Geometry: final body of the model. Coordinates: model frame, mm. A direction names the side the tool comes from. Give positions to 0.01 mm unless a question says otherwise; leave off trailing zeros. Order: outer loops, then holes, each group sorted by start corner. A loop starts at its lowest first (then second) coordinate and runs counter-clockwise, first axis right, second up. Notation, with made-up numbers: (43.25, 72.25) - (72.25, 72.25) arc R28 ccw to (72.25, 90.25) - close; hole circle Ø9 at (-23.75, 35). An arc over 180 degrees is marked (long way). One line per question, with ' | ' between items. Start each with the question number.
from build123d import *

# Parameters (mm, degrees)
SKETCH7_W           = 100
SKETCH7_H           = 14.5
BOSS_EXTRUDE1_DEPTH = 16.5
SKETCH8_R           = 4.75
CUT_EXTRUDE2_DEPTH  = 16
CUT_EXTRUDE3_START  = -2
SKETCH9_W           = 27
SKETCH9_H           = 27
CUT_EXTRUDE3_DEPTH  = 2
CUT_EXTRUDE4_DEPTH  = 2
FILLET1_R           = 3
FILLET2_R           = 3
FILLET3_R           = 0.3


with BuildPart() as part:
    # Sketch7 → Boss-Extrude1 (new body)
    with BuildSketch(Plane(origin=(0, 0, 0), x_dir=(0, 1, 0), z_dir=(0, 0, 1))):
        Rectangle(SKETCH7_W, SKETCH7_H)
    extrude(amount=BOSS_EXTRUDE1_DEPTH)

    # Sketch8 → Cut-Extrude2 (cut)
    with BuildSketch(Plane(origin=(0, 0, 16.5), x_dir=(0, -1, 0), z_dir=(0, 0, 1))):
        with Locations(Location((0, 0, 0), (0, 0, 90))):
            Circle(SKETCH8_R)
    extrude(amount=-CUT_EXTRUDE2_DEPTH, mode=Mode.SUBTRACT)

    # Sketch9 → Cut-Extrude3 (cut)
    with BuildSketch(Plane.XY.offset(16.5).offset(CUT_EXTRUDE3_START)):
        with Locations((0, -31.55)):
            Rectangle(SKETCH9_W, SKETCH9_H)
    cut_extrude3 = extrude(amount=-CUT_EXTRUDE3_DEPTH, mode=Mode.SUBTRACT)

    # Sketch10 → Cut-Extrude4 (cut)
    with BuildSketch(Plane.XY.offset(16.5)):
        with BuildLine():
            Line((0, -24.55), (-7.25, -24.55))
            Line((-7.25, -24.55), (-7.25, -38.55))
            Line((-7.25, -38.55), (0, -38.55))
            ThreePointArc((0, -38.55), (7, -31.55), (0, -24.55))
        make_face()
    cut_extrude4 = extrude(amount=-CUT_EXTRUDE4_DEPTH, mode=Mode.SUBTRACT)

    # Mirror1: Cut-Extrude3 across plane
    add(cut_extrude3.mirror(Plane.ZX), mode=Mode.SUBTRACT)

    # Mirror2: Cut-Extrude4 across plane
    add(cut_extrude4.mirror(Plane.ZX), mode=Mode.SUBTRACT)

    # Fillet1
    fillet1_edges = [part.edges().sort_by_distance(p)[0] for p in [
        (-7.25, 0, 0),
    ]]
    fillet(fillet1_edges, radius=FILLET1_R)

    # Fillet2
    fillet2_edges = [part.edges().sort_by_distance(p)[0] for p in [
        (7.25, 0, 0),
    ]]
    fillet(fillet2_edges, radius=FILLET2_R)

    # Fillet3
    fillet3_edges = [part.edges().sort_by_distance(p)[0] for p in [
        (-4.75, 0, 16.5),
    ]]
    fillet(fillet3_edges, radius=FILLET3_R)


solid = part.part
(1) Cut plane C-C, the plane z = 10.5. Return the cut outline in (x, y).
(2) Cut plane B-B, the plane y = -31.55. Return the cut outline in (x, z), plus the area to 3 significant figures.
(3) Cut plane D-D, the plane x = 6. Return the cut outline in (y, z).
(4) Pull-direction query (Y, two-part tool) for faces 4 (the flat face through (-7.25, -1, 10)), 5 (the flat face through (0, 50, 8)), 6 (the flat face through (5, -25, 14.5)); classes: +Y half, -Y half, draft (parallel to the pull), parting line (faces both ways), or undercut.
(5) Material intervals for line 1 along Y through (x, z) = (0, 12.75); line 2 along Y through (x, z) = (0.25, 14.75); line 3 along Y through (x, z) = (0, 10.75), sorted ascending. Write a range as from..to.
(6) Contact query for a flat-ended pin moving along its axis: P1, Ø4.5, axis at x = 3.5, y = 27, coming from the +Z side. Output: stop coordinate, or through.
(7) Access query for faces 1 (the cylindrical face through (6.35, 0.7, 0.86)), 2 (the flat face through (-4, -38.55, 16)), 3 (the flat face through (5, 25, 14.5)). Directions: +Z, -Z, +X, -X, +Y, -Y. A direction counts if a zero-diameter tool reaches every point of the face in a straight line with its end or side. Return the directions, or none.
(8) Cut plane A-A, the plane y = 41. Return the cut outline in (x, z), plus the area to 3 significant figures.
Results are:
1) outline: (-7.25, -50) - (7.25, -50) - (7.25, 50) - (-7.25, 50) - close; hole circle Ø9.5 at (0, 0)
2) outline: (-7.25, 3) arc R3 ccw to (-4.25, 0) - (4.25, 0) arc R3 ccw to (7.25, 3) - (7.25, 12.5) - (-7.25, 12.5) - close; (7, 14.5) - (7.25, 14.5) - (7.25, 16.5) - (7, 16.5) - close | area: 178 mm2
3) outline: (-50, 0.56) - (50, 0.56) - (50, 16.5) - (35.16, 16.5) - (35.16, 14.5) - (45.05, 14.5) - (45.05, 12.5) - (18.05, 12.5) - (18.05, 14.5) - (27.94, 14.5) - (27.94, 16.5) - (-27.94, 16.5) - (-27.94, 14.5) - (-18.05, 14.5) - (-18.05, 12.5) - (-45.05, 12.5) - (-45.05, 14.5) - (-35.16, 14.5) - (-35.16, 16.5) - (-50, 16.5) - close
4) face 4: draft | face 5: +Y half | face 6: undercut
5) line 1: -50..-45.05, -18.05..-4.75, 4.75..18.05, 45.05..50 | line 2: -50..-38.55, -24.55..-4.74, 4.74..24.55, 38.55..50 | line 3: -50..-4.75, 4.75..50
6) P1: z = 16.5
7) face 1: -Z, +X, +Y, -Y | face 2: +Z, -X | face 3: +X, -X
8) outline: (-7.25, 3) arc R3 ccw to (-4.25, 0) - (4.25, 0) arc R3 ccw to (7.25, 3) - (7.25, 12.5) - (-7.25, 12.5) - close; (-7.25, 14.5) - (7.25, 14.5) - (7.25, 16.5) - (-7.25, 16.5) - close | area: 206 mm2
